from build123d import *

# Parameters (mm, degrees)
BOSS_EXTRUDE1_DEPTH  = 1
FILLET1_R            = 1
CUT_EXTRUDE1_START   = -3
CUT_EXTRUDE1_DEPTH   = 4
FILLET2_R            = 1
FILLET2_OF_MIRROR1_R = 1


with BuildPart() as part:
    # Sketch1 → Boss-Extrude1 (new body, symmetric)
    with BuildSketch(Plane(origin=(0, 0, 0), x_dir=(1, 0, 0), z_dir=(0, 1, 0))):
        Polygon((12.7, 12.7), (15.875, 12.7), (15.875, 15.875), (-15.875, 15.875), (-15.875, 12.7), (-12.7, 12.7), (-12.7, -12.7), (-15.875, -12.7), (-15.875, -15.875), (15.875, -15.875), (15.875, -12.7), (12.7, -12.7), align=None)
    extrude(amount=BOSS_EXTRUDE1_DEPTH, both=True)

    # Fillet1
    fillet1_edges = [part.edges().sort_by_distance(p)[0] for p in [
        (12.7, 0, 12.7),
        (15.875, 0, 12.7),
        (15.875, 0, 15.875),
        (-15.875, 0, 15.875),
        (-15.875, 0, 12.7),
        (-12.7, 0, 12.7),
        (-12.7, 0, -12.7),
        (-15.875, 0, -12.7),
        (-15.875, 0, -15.875),
        (15.875, 0, -15.875),
        (15.875, 0, -12.7),
        (12.7, 0, -12.7),
    ]]
    fillet(fillet1_edges, radius=FILLET1_R)

    # Sketch2 → Cut-Extrude1 (cut)
    with BuildSketch(Plane(origin=(0, 1, 0), x_dir=(1, 0, 0), z_dir=(0, 1, 0)).offset(CUT_EXTRUDE1_START)):
        Polygon((-8.73125, 15.875), (-4.7625, 11.750554014), (-7.14375, 15.875), align=None)
    cut_extrude1 = extrude(amount=CUT_EXTRUDE1_DEPTH, mode=Mode.SUBTRACT)

    # Fillet2
    fillet2_edges = [part.edges().sort_by_distance(p)[0] for p in [
        (-7.14375, 0, -15.875),
        (-8.73125, 0, -15.875),
    ]]
    fillet(fillet2_edges, radius=FILLET2_R)

    # Mirror1: Cut-Extrude1 across plane
    add(cut_extrude1.mirror(Plane(origin=(0, 0, 0), x_dir=(0, 0, 1), z_dir=(1, 0, 0))), mode=Mode.SUBTRACT)

    # Fillet2 of Mirror1
    fillet2_of_mirror1_edges = [part.edges().sort_by_distance(p)[0] for p in [
        (7.14375, 0, -15.875),
        (8.73125, 0, -15.875),
    ]]
    fillet(fillet2_of_mirror1_edges, radius=FILLET2_OF_MIRROR1_R)


solid = part.part
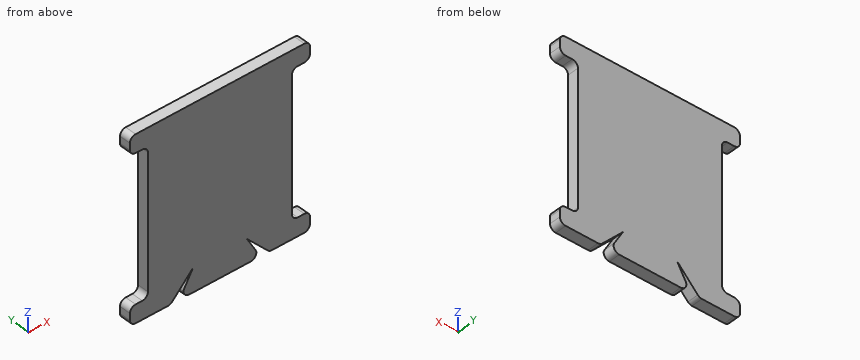
For this review, take the finished solid that the model builds, in its own axes (mm). Give positions to 0.01 mm unless a question says otherwise; leave off trailing zeros. Order: outer loops, then holes, each group sorted by start corner. A loop starts at its lowest first (then second) coordinate and runs counter-clockwise, first axis right, second up. Notation, with made-up numbers: (3, -13) -> (59, -13) arc R6 cw to (59, -8) -> close; hole circle Ø5 at (39.25, -14). An arc over 180 degrees is marked (long way). Write item = value, one per line.
1) We need section C-C, the plane x = -7. Give the boundary of the cut face in (y, z) (3 decimals), and give its area (3 significant figures).
Findings:
outline = (-1, -14.076) -> (1, -14.076) -> (1, 15.875) -> (-1, 15.875) -> close
area = 59.9 mm^2
2) To check wall thickness, follow L1, parallel to X at y = 0, z = 2; L2, parallel to Z at x = 7.5, y = 0.7 (3 decimals); L3, parallel to Z at x = -7, y = 0.5 (3 decimals). State the ranges of each line that lie inside material, in increasing order. Write a range as from..to.
Findings:
L1 = -12.7..12.7
L2 = -14.595..15.875
L3 = -14.076..15.875
3) We need section B-B, the plane z = 11. Give the boundary of the cut face in (x, y).
Findings:
outline = (-12.7, -1) -> (12.7, -1) -> (12.7, 1) -> (-12.7, 1) -> close
4) Insertion check: pin 1 (1 mm diameter, centred on y = 0, z = -8.5, fed in from -X). The pin has a flat end and moves straight along its axis. Give the tip position at first contact, or say it passes through.
Findings:
pin_1 = -12.7
